Part model, mm, in its own coordinate system. A direction names the side the tool comes from. Round coordinates to 2 decimals unless told otherwise and drop trailing zeros. Order: outer loops, then holes, each group sorted by start corner. A loop starts at its lowest first (then second) coordinate and runs counter-clockwise, first axis right, second up. Notation, with made-up numbers: M 23,44 L 65,44 A23 cw 65,53 Z; hole C -38.75,62 d11. An arc over 180 degrees is marked long. Write each question's results on one line, items separated by ' | '. Start each with the question number.
1. Band-saw the part on A-A, the plane y = 10. List the corners of the cut face in (x, z) (3 decimals).
2. Two-plate mould, pull along Y, no slides. Class faces 1 (the face through (-46.98, 3.43, 12.52)), 2 (the face through (1, 15.405, 33)), 3 (the face through (0, -1, 66.04)), 4 (the face through (0.308, 15.951, 0.764)): +Y half, -Y half, draft (parallel to the pull), parting line (faces both ways), or undercut.
3. Band-saw the part on D-D, the plane y = 0.5. List the corners of the cut face in (x, z) (3 decimals).
4. Probe L1, parallel to Z at x = -40.5, y = 14; L2, parallel to X at y = -1, z = 15 (3 decimals); L3, parallel to Y at x = 43.5, z = 48. List the from-to ranges inside material, lowest first. Write a range as [from, to].
5. Band-saw the part on B-B, the plane x = -27. List the corners of the cut face in (y, z) (3 decimals), then the cut area to 3 significant figures.
6. Band-saw the part on C-C, the plane z = 32.5. List the corners of the cut face in (x, y) (3 decimals).
7. Drop flat-ended pins along their axis: pin 1 Ø3 at (y, z) = (-1.5, 55.5) entering from +X (3 decimals); pin 2 Ø1.5 at (x, y) = (25, -5.5) entering from -Z; pin 3 Ø6 at (x, z) = (21, 17.5) entering from -Y. Give the stop position or say it passes through.
8. Which spindle directions (+Z, -Z, +X, -X, +Y, -Y) get a long thin tool onto all of the face, cutting with end or side? Do faces 5 (the face through (-47.625, -1, 33)), 6 (the face through (0, 0, 64.77)). Say none if no direction does.
Autodesk Inventor part; units mm, degrees
ref_plane "YZ Plane" through (0, 0, 0) normal (1, 0, 0) x (0, 1, 0)
ref_plane "XZ Plane" through (0, 0, 0) normal (0, 1, 0) x (-1, 0, 0)
ref_plane "XY Plane" through (0, 0, 0) normal (0, 0, 1) x (1, 0, 0)
sketch "Sketch1" plane through (0, 0, 0) normal (0, 0, 1) x (1, 0, 0)
  line L0 (-47.625, -16.6751) -> (47.625, -16.6751)
  line L1 (47.625, -16.6751) -> (47.625, 16.6751)
  line L2 (47.625, 16.6751) -> (-47.625, 16.6751)
  line L3 (-47.625, 16.6751) -> (-47.625, -16.6751)
  line L4 (-47.625, -16.6751) -> (47.625, 16.6751) construction
  line L5 (47.625, -16.6751) -> (-47.625, 16.6751) construction
  point P0 (0, 0)
  dimension "d0" = 95.25
  dimension "d1" = 33.3502
extrude "Extrusion1" add sketch "Sketch1" along normal blind 66.04
shell "Shell1" thickness 1.27 removed faces 2 at (-15.875, -16.6751, 44.0267) at (47.625, -5.5584, 44.0267)
sketch "Sketch2" plane through (-46.355, -16.6751, 1.27) normal (1, 0, 0) x (0, 0, -1)
  line L0 (0, 32.0802) -> (0, 0)
  line L1 (0, 0) -> (-63.5, 0)
  circle A0 centre (-14.351, 19.1262) radius 3.2512
  point P0 (1.27, 16.6751)
  dimension "d5" = 14.351
  dimension "d6" = 19.1262
  dimension "d7" = 6.5024
extrude "Extrusion2" cut sketch "Sketch2" against normal up to surface (1.27 mm away)
fillet "Fillet1" radius 2.54 5 edges at (0, 16.6751, 66.04) (-47.625, 16.6751, 33.02) (0, 16.6751, 0) (-47.625, 0, 0) (-47.625, 0, 66.04)
fillet "Fillet2" radius 0.635 5 edges at (47.625, -1.27, 0) (47.625, 15.9312, 0.7439) (47.625, 16.6751, 33.02) (47.625, 15.9312, 65.2961) (47.625, -1.27, 66.04)
fillet "Fillet3" radius 0.635 9 edges at (47.439, -16.6751, 65.854) (47.625, -16.6751, 65.0875) (-46.8811, -16.6751, 65.2961) (-47.625, -16.6751, 33.02) (-46.8811, -16.6751, 0.7439) (0.9525, -16.6751, 0) (47.439, -16.6751, 0.186) (47.625, -16.6751, 0.9525) (0.9525, -16.6751, 66.04)
properties part number "ECG_cover"
Solution:
1) outline: M -47.625,2.54 A2.54 ccw -45.085,0 L 46.99,0 A0.635 ccw 47.625,0.635 L 47.625,1.27 L -46.355,1.27 L -46.355,64.77 L 47.625,64.77 L 47.625,65.405 A0.635 ccw 46.99,66.04 L -45.085,66.04 A2.54 ccw -47.625,63.5 Z
2) face 1: undercut | face 2: -Y half | face 3: draft | face 4: +Y half
3) outline: M -47.625,2.54 A2.54 ccw -45.085,0 L 46.99,0 A0.635 ccw 47.625,0.635 L 47.625,1.27 L -46.355,1.27 L -46.355,13.02 L -47.625,13.02 Z; M -47.625,18.222 L -46.355,18.222 L -46.355,64.77 L 47.625,64.77 L 47.625,65.405 A0.635 ccw 46.99,66.04 L -45.085,66.04 A2.54 ccw -47.625,63.5 Z
4) L1: [0, 1.27], [64.77, 66.04] | L2: [-47.625, -46.355] | L3: [15.41, 16.68]
5) outline: M -16.675,0.635 A0.635 ccw -16.04,0 L 14.135,0 A2.54 ccw 16.675,2.54 L 16.675,63.5 A2.54 ccw 14.135,66.04 L -16.04,66.04 A0.635 ccw -16.675,65.405 L -16.675,64.77 L 15.405,64.77 L 15.405,1.27 L -16.675,1.27 Z | area: 162 mm^2
6) outline: M -47.625,-16.04 A0.635 ccw -46.99,-16.675 L -46.355,-16.675 L -46.355,15.405 L 47.625,15.405 L 47.625,16.04 A0.635 ccw 46.99,16.675 L -45.085,16.675 A2.54 ccw -47.625,14.135 Z
7) pin 1: x = -46.355 | pin 2: z = 0 | pin 3: y = 15.41
8) face 5: +Z, -Z, -X, +Y, -Y | face 6: +X, -Y
